```python
from build123d import *

# Parameters (mm, degrees)
F0_W     = 8
F0_H     = 15
F1_DEPTH = 15
F1_TAPER = 3
F2_R     = 1.7138833108
F3_DEPTH = 5
F4_R     = 1.5
F5_DEPTH = 1
F6_R     = 1.5
F7_DEPTH = 1
F8_R     = 1


with BuildPart() as f1:
    # F0 (on Top) → F1 (new body)
    with BuildSketch(Plane.XY):
        Rectangle(F0_W, F0_H)
    extrude(amount=F1_DEPTH, taper=F1_TAPER)

    # F2 (on face) → F3 (join)
    with BuildSketch(Plane.XY.offset(15)):
        Circle(F2_R)
    extrude(amount=F3_DEPTH)

    # F4 (on face) → F5 (cut)
    with BuildSketch(Plane(origin=(0, 7.4794571076, 0.3919817373), x_dir=(-1, 0, 0), z_dir=(0, 0.9986295348, 0.0523359562))):
        with Locations((0, 9.6280655181)):
            Circle(F4_R)
    extrude(amount=-F5_DEPTH, mode=Mode.SUBTRACT)

    # F6 (on face) → F7 (cut)
    with BuildSketch(Plane(origin=(0, -7.4794571076, 0.3919817373), x_dir=(1, 0, 0), z_dir=(0, -0.9986295348, 0.0523359562))):
        with Locations((0, 9.6280655181)):
            Circle(F6_R)
    extrude(amount=-F7_DEPTH, mode=Mode.SUBTRACT)

    # F8
    f8_edges = [f1.edges().sort_by_distance(p)[0] for p in [
        (-3.213883, 0, 15),
        (-3.606942, 7.106942, 7.5),
        (-3.606942, -7.106942, 7.5),
        (3.213883, 0, 15),
        (3.606942, -7.106942, 7.5),
        (3.606942, 7.106942, 7.5),
    ]]
    fillet(f8_edges, radius=F8_R)


solid = f1.part
```
Geometry: final body of the model. Coordinates: model frame, mm. Coordinates: 2 decimals unless noted, no trailing zeros. Write each loop counter-clockwise with the first axis right and the second up, starting at its lowest first coordinate (ties: lowest second). Pieces come first, ordered by that corner, then holes. Notation, with made-up numbers: M 52,35.5 L 104,35.5 A22 cw 104,53.5 Z; hole C 21.25,12.5 d4. An arc over 180 degrees is marked long. Answer as CSV lines item,"result". Start each with the question number.
Q1. Cut plane C-C on z = 15.75. Return the cut outline in (x, y), then the cut area to 3 significant figures.
Q2. Mould query, pull axis Z, two halves, no side actions, for faces 1 (the flat face through (3.637, 0.091, 6.928)), 2 (the cylindrical face through (-0.22, 1.7, 17.46)), 3 (the flat face through (-0.021, -5.976, 9.975)). Classes: released by +Z, released by -Z, zero draft, split by the parting line, or undercut.
Q3. Cut plane A-A on x = 1. Return the cut outline in (y, z).
Q4. Line query: line 1 (Z direction, x = -1.25, y = -1.25); line 2 (Z direction, x = 0.25, y = 6.5); line 3 (X direction, y = 3.25, z = 13). Output: solid intervals per line, ascending. Write a range as from..to.
Q5. Cut plane B-B on y = 0. Return the cut outline in (x, z).
Q6. Pin query (flat end, axial travel): P1, Ø1, axis at y = 5, z = 10.5, coming from the -X side; P2, Ø2, axis at x = -2.5, y = -4, coming from the +Z side; P3, Ø1.5, axis at x = 2.5, z = 3.5, coming from the +Y side. Return the tip coordinate at first contact, or that it passes through.
Q7. Cut plane D-D on x = -1.25. Return the cut outline in (y, z).
Findings below:
1,outline,"C 0,0 d3.43"
1,area,"9.23 mm2"
2,face 1,"released by +Z"
2,face 2,"zero draft"
2,face 3,"undercut"
3,outline,"M -7.5,0 L 7.5,0 L 7.03,8.89 L 6.04,8.84 L 5.92,11.07 L 6.92,11.12 L 6.71,15 L 1.39,15 L 1.39,20 L -1.39,20 L -1.39,15 L -6.71,15 L -6.92,11.12 L -5.92,11.07 L -6.04,8.84 L -7.03,8.89 Z"
4,line 1,"z = 0..15"
4,line 2,"z = 0..8.5, 11.46..15"
4,line 3,"x = -3.32..3.32"
5,outline,"M -4,0 L 4,0 L 3.26,14.05 A1 ccw 2.26,15 L 1.71,15 L 1.71,20 L -1.71,20 L -1.71,15 L -2.26,15 A1 ccw -3.26,14.05 Z"
6,P1,"stops at x = -3.48"
6,P2,"stops at z = 15"
6,P3,"stops at y = 7.36"
7,outline,"M -7.5,0 L 7.5,0 L 7.02,9.18 L 6.02,9.13 L 5.93,10.78 L 6.93,10.83 L 6.71,15 L 1.17,15 L 1.17,20 L -1.17,20 L -1.17,15 L -6.71,15 L -6.93,10.83 L -5.93,10.78 L -6.02,9.13 L -7.02,9.18 Z"
